Geometry check sheet. Reference: the model listing, model coordinates, mm. A direction names the side the tool comes from. Coordinates: 2 decimals unless noted, no trailing zeros. Loops run counter-clockwise (first coordinate to the right, second up) from the corner with the lowest first, then second, coordinate; pieces in that order, holes last.
from build123d import *

# Parameters (mm, degrees)
BOX001_W     = 70
BOX001_H     = 49
BOX001_DEPTH = 9
BOX_W        = 70
BOX_H        = 53
BOX_DEPTH    = 2
SKETCH_R     = 2
POCKET_DEPTH = 9.001


with BuildPart() as cube001:
    # Box001 → Box001 (new body)
    with BuildSketch(Plane.XY):
        with Locations((35, 24.5)):
            Rectangle(BOX001_W, BOX001_H)
    extrude(amount=BOX001_DEPTH)


with BuildPart() as pocket:
    # Box → Box (new body)
    with BuildSketch(Plane.XY):
        with Locations((35, 26.5)):
            Rectangle(BOX_W, BOX_H)
    extrude(amount=BOX_DEPTH)

    # Fusion: union Cube001
    add(cube001.part)

    # Sketch → Pocket (cut, through all)
    with BuildSketch(Plane.XY.offset(9)):
        with Locations((13, 14)):
            Circle(SKETCH_R)
        with Locations((13, 35)):
            Circle(SKETCH_R)
        with Locations((57, 35)):
            Circle(SKETCH_R)
        with Locations((57, 14)):
            Circle(SKETCH_R)
    extrude(amount=-POCKET_DEPTH, mode=Mode.SUBTRACT)


solid = pocket.part
(1) Access from +Z, -Z, +X, -X, +Y, -Y to the whole of each face (thin tool, end or side, straight path). Record for faces 1 (the flat face through (35, 51, 2)), 2 (the flat face through (0, 26, 4)).
Findings:
face 1: +Z, +X, -X, +Y
face 2: +Z, -Z, -X, +Y, -Y
(2) Sectioned sample at B-B on x = 13. Record the cut outline in (y, z), and give its area (3 significant figures).
Findings:
outline: (0, 0) - (12, 0) - (12, 9) - (0, 9) - close; (16, 0) - (33, 0) - (33, 9) - (16, 9) - close; (37, 0) - (53, 0) - (53, 2) - (49, 2) - (49, 9) - (37, 9) - close
area: 377 mm2
(3) Gauge pin test, flat ends, axial feed: pin 1 Ø4 at (x, z) = (21, 5) entering from +Y; pin 2 Ø1.2 at (x, y) = (31.5, 50.5) entering from +Z. Record the tip position at first contact, or that the pin passes through.
Findings:
pin 1: stops at y = 49
pin 2: stops at z = 2
(4) Scan lines: L1, parallel to Y at x = 13, z = 6; L2, parallel to Y at x = 23.5, z = 6.25; L3, parallel to Z at x = 66.5, y = 50. Record each from-to range of solid material in increasing order.
Findings:
L1: y = 0 to 12, 16 to 33, 37 to 49
L2: y = 0 to 49
L3: z = 0 to 2
(5) Sectioned sample at D-D on x = 25. Record the cut outline in (y, z).
Findings:
outline: (0, 0) - (53, 0) - (53, 2) - (49, 2) - (49, 9) - (0, 9) - close
(6) Sectioned sample at C-C on z = 4.75. Record the cut outline in (x, y), and give its area (3 significant figures).
Findings:
outline: (0, 0) - (70, 0) - (70, 49) - (0, 49) - close; hole circle Ø4 at (13, 14); hole circle Ø4 at (13, 35); hole circle Ø4 at (57, 14); hole circle Ø4 at (57, 35)
area: 3,380 mm2
(7) Sectioned sample at A-A on y = 35. Record the cut outline in (x, z).
Findings:
outline: (0, 0) - (11, 0) - (11, 9) - (0, 9) - close; (15, 0) - (55, 0) - (55, 9) - (15, 9) - close; (59, 0) - (70, 0) - (70, 9) - (59, 9) - close
(8) Draft check along Y on faces 3 (the flat face through (35, 27, 0)), 4 (the cylindrical face through (11.526, 15.352, 4.563)), 5 (the flat face through (35, 53, 1)). Enter one of: +Y half, -Y half, draft (parallel to the pull), parting line (faces both ways), or undercut.
Findings:
face 3: draft
face 4: undercut
face 5: +Y half
